Read the model definition and answer for the solid it produces. Units are mm, in the model's axes. A direction names the side the tool comes from. Give positions to 0.01 mm unless a question says otherwise; leave off trailing zeros. Order: outer loops, then holes, each group sorted by start corner. A loop starts at its lowest first (then second) coordinate and runs counter-clockwise, first axis right, second up.
Item 1: A cutting plane is placed at B-B (x = -11.5). Write down the section's boundary in (y, z), plus the area to 3 significant figures.
Item 2: A cutting plane is placed at A-A (y = -22). Write down the section's boundary in (x, z), plus the area to 3 significant figures.
Item 3: Given pin 1 Ø1 at (y, z) = (-21, 22) entering from +X; pin 2 Ø2.5 at (x, y) = (-15, -22.5) entering from -Z; pin 3 Ø3 at (y, z) = (-24.5, 21) entering from -X, each flat-ended and moving along its own axis, determine where each tip first touches the part or whether it passes through.
Item 4: A cutting plane is placed at C-C (z = 24). Write down the section's boundary in (x, y), plus the area to 3 significant figures.
Item 5: Find the intervals of material crossed by line 1 along Z through (x, y) = (-26, -21.15); line 2 along Z through (x, y) = (14, -22.45); line 3 along X through (y, z) = (-23.25, 29.5), in increasing order.
Item 6: Which of the six approach directions +Z, -Z, +X, -X, +Y, -Y give full straight-line access (tool end or side, diameter ignored) to faces 1 (the face through (7.545, -22, 26)), 2 (the face through (8, -25, 31)), 3 (the face through (27, -22, 10.698))?
from build123d import *

# Parameters (mm, degrees)
F1_DEPTH = 25
F2_DEPTH = 20
F3_DEPTH = 15


with BuildPart() as f1:
    # F0 (on Front) → F1 (new body)
    with BuildSketch(Plane.XZ):
        Polygon((7.5449606204, 50.6978626826), (-37.4550393796, 50.6978626826), (-37.4550393796, 45.6978626826), (7.5449606204, 45.6978626826), (7.5449606204, 5.6978626826), (12.5449606204, 5.6978626826), (27.5449606204, 5.6978626826), (27.5449606204, 10.6978626826), (12.5449606204, 10.6978626826), (12.5449606204, 50.6978626826), align=None)
    extrude(amount=F1_DEPTH)

    # F2 (cut): a face of the model
    f2_faces = [f1.faces().sort_by_distance(p)[0] for p in [
        (-36.6644699645, 0, 48.1978626826),
    ]]
    extrude(f2_faces, amount=-F2_DEPTH, mode=Mode.SUBTRACT)

    # F3 (add): a face of the model
    f3_faces = [f1.faces().sort_by_distance(p)[0] for p in [
        (27.5449606204, -22.5, 8.1978626826),
    ]]
    extrude(f3_faces, amount=F3_DEPTH)


solid = f1.part
Response values:
1. outline: (-25, 45.7) - (-20, 45.7) - (-20, 50.7) - (-25, 50.7) - close
1. area: 25.0 mm2
2. outline: (-37.46, 45.7) - (7.54, 45.7) - (7.54, 5.7) - (42.54, 5.7) - (42.54, 10.7) - (12.54, 10.7) - (12.54, 50.7) - (-37.46, 50.7) - close
2. area: 600 mm2
3. pin 1: stops at x = 12.54
3. pin 2: stops at z = 45.7
3. pin 3: stops at x = 7.54
4. outline: (7.54, -25) - (12.54, -25) - (12.54, -20) - (7.54, -20) - close
4. area: 25.0 mm2
5. line 1: z = 45.7 to 50.7
5. line 2: z = 5.7 to 10.7
5. line 3: x = 7.54 to 12.54
6. face 1: -Z, -X, +Y, -Y
6. face 2: +Z, -Z, +X, -X, -Y
6. face 3: +Z, +X, +Y, -Y
